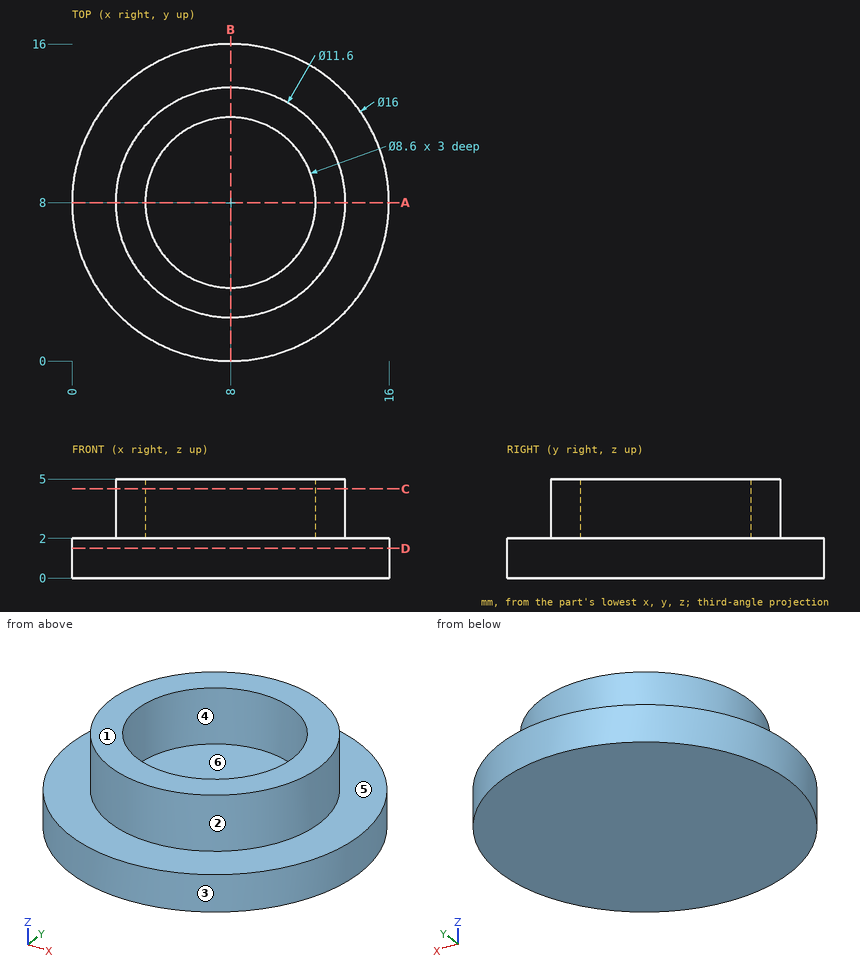
Job drawing, mm, ordinate dimensions from the low corner. One solid piece. A direction names the side the tool comes from. Round coordinates to 2 decimals unless told otherwise and drop trailing zeros. Write each loop counter-clockwise with the first axis right and the second up, starting at its lowest first coordinate (ties: lowest second). Pieces come first, ordered by that corner, then holes. Notation, with made-up numbers: (82.5, -32) -> (112.5, -32) arc R7 ccw to (112.5, -26) -> close; hole circle Ø2 at (66, 0.25). An arc over 180 degrees is marked (long way). Answer as CSV lines item,"result".
1. Slice it at A-A, the plane y = 8. List the corners of the cut face in (x, z).
Resolved:
outline,"(0, 0) -> (16, 0) -> (16, 2) -> (13.8, 2) -> (13.8, 5) -> (12.3, 5) -> (12.3, 2) -> (3.7, 2) -> (3.7, 5) -> (2.2, 5) -> (2.2, 2) -> (0, 2) -> close"
2. Slice it at C-C, the plane z = 4.5. List the corners of the cut face in (x, y).
Resolved:
outline,"circle Ø11.6 at (8, 8); hole circle Ø8.6 at (8, 8)"
3. Drill centre lines: line 1 (Y direction, x = 8, z = 3.55); line 2 (Z direction, x = 9.5, y = 8); line 3 (X direction, y = 8.75, z = 3.65). Where is each one in solid material? Low to high.
Resolved:
line 1,"2.2 to 3.7, 12.3 to 13.8"
line 2,"0 to 2"
line 3,"2.25 to 3.77, 12.23 to 13.75"
4. Tool access for the marked faces 1 and 2: list every direction of +Z, -Z, +X, -X, +Y, -Y with a clear straight run to the whole face (end or side of a thin tool).
Resolved:
face 1,"+Z, +X, -X, +Y, -Y"
face 2,"+Z"
5. Mould opens along Y. For the marked faces 3, 4, 5 and 6 say: +Y half, -Y half, draft (parallel to the pull), parting line (faces both ways), or undercut.
Resolved:
face 3,"parting line"
face 4,"undercut"
face 5,"draft"
face 6,"undercut"
6. Pin check, flat tips, straight feed: pin 1 Ø5 at (x, y) = (6.5, 12.5) entering from -Z; pin 2 Ø1 at (x, z) = (8.5, 3) entering from -Y; pin 3 Ø1.5 at (y, z) = (11.5, 1.5) entering from +X; pin 4 Ø2.5 at (x, y) = (6.5, 6) entering from +Z. Stop position of each tip, or through.
Resolved:
pin 1,"z = 0"
pin 2,"y = 2.2"
pin 3,"x = 15.51"
pin 4,"z = 2"
7. Slice it at D-D, the plane z = 1.5. List the corners of the cut face in (x, y), plus the area to 3 significant figures.
Resolved:
outline,"circle Ø16 at (8, 8)"
area,"201 mm²"
